Input: part model. Units: mm. Frame: model coordinates. Round coordinates to 2 decimals unless told otherwise and drop trailing zeros. Order: outer loops, then holes, each group sorted by start corner. A loop starts at its lowest first (then second) coordinate and runs counter-clockwise, first axis right, second up.
Item 1: Line query: L1, parallel to X at y = -3, z = 2.2; L2, parallel to Y at x = 12, z = 2.9; L3, parallel to X at y = -3.3, z = 2. Output: solid intervals per line, ascending.
Item 2: Cut plane A-A on x = 3.75. Output: boundary loops of the cut face in (y, z).
Item 3: Cut plane C-C on z = 3.25. Give the number of separate pieces and of enclosed holes in the cut face, then the cut area to 3 significant figures.
Item 4: Cut plane B-B on y = -1.9. Output: boundary loops of the cut face in (x, z).
Item 5: Mould query, pull axis Y, two halves, no side actions, for faces 1 (the cylindrical face through (10.55, -2.94, 1.97)), 2 (the flat face through (7, -6, 2)), 3 (the flat face through (7, 0, 2)). Classes: released by +Y, released by -Y, zero draft, split by the parting line, or undercut.
Item 6: First-contact query: pin 1 (1.5 mm diameter, centred on y = -5, z = 1.5, fed in from +X); pin 2 (1.5 mm diameter, centred on y = -1.5, z = 1.5, fed in from +X); pin 3 (1.7 mm diameter, centred on x = 12, y = -3, fed in from +Z). Flat tips, straight axial feed; report the tip coordinate or a pass-through.
Item 7: Cut plane D-D on y = -3.6. Output: boundary loops of the cut face in (x, z).
```python
from build123d import *

# Parameters (mm, degrees)
SKETCH1_W               = 15
SKETCH1_H               = 6
BOSS_EXTRUDE1_DEPTH     = 4
CUT_EXTRUDE1_DEPTH      = 17.643316977
CUT_EXTRUDE1_DEPTH_BACK = 17.643316977
SKETCH2_R               = 0.9
SKETCH2_R_2             = 1.45
FILLET1_R               = 3


with BuildPart() as part:
    # Sketch1 → Boss-Extrude1 (new body)
    with BuildSketch(Plane.XY):
        with Locations((7.5, -3)):
            Rectangle(SKETCH1_W, SKETCH1_H)
    extrude(amount=BOSS_EXTRUDE1_DEPTH)

    # Sketch2 → Cut-Extrude1 (cut, two sides: drawn at the far end of the back side and taken through both)
    with BuildSketch(Plane.XY.offset(4).offset(-CUT_EXTRUDE1_DEPTH_BACK)):
        with Locations((3, -3)):
            Circle(SKETCH2_R)
        with Locations((12, -3)):
            Circle(SKETCH2_R_2)
    extrude(amount=CUT_EXTRUDE1_DEPTH + CUT_EXTRUDE1_DEPTH_BACK, mode=Mode.SUBTRACT)

    # Fillet1
    fillet1_edges = [part.edges().sort_by_distance(p)[0] for p in [
        (15, -6, 2),
        (15, 0, 2),
        (0, -6, 2),
        (0, 0, 2),
    ]]
    fillet(fillet1_edges, radius=FILLET1_R - 0.0001)  # a hair under: the kernel refuses the full size


solid = part.part
```
From the geometry:
1. L1: x = 0 to 2.1, 3.9 to 10.55, 13.45 to 15
1. L2: y = -6 to -4.45, -1.55 to 0
1. L3: x = 0.02 to 2.15, 3.85 to 10.58, 13.42 to 14.98
2. outline: (-6, 0) - (-3.5, 0) - (-3.5, 4) - (-6, 4) - close; (-2.5, 0) - (0, 0) - (0, 4) - (-2.5, 4) - close
3. separate pieces: 1
3. enclosed holes: 2
3. area: 73.1 mm2
4. outline: (0.21, 0) - (11.06, 0) - (11.06, 4) - (0.21, 4) - close; (12.94, 0) - (14.79, 0) - (14.79, 4) - (12.94, 4) - close
5. face 1: undercut
5. face 2: released by -Y
5. face 3: released by +Y
6. pin 1: stops at x = 14.73
6. pin 2: stops at x = 14.9
6. pin 3: passes through
7. outline: (0.06, 0) - (2.33, 0) - (2.33, 4) - (0.06, 4) - close; (3.67, 0) - (10.68, 0) - (10.68, 4) - (3.67, 4) - close; (13.32, 0) - (14.94, 0) - (14.94, 4) - (13.32, 4) - close
